```python
from build123d import *

# Parameters (mm, degrees)
BOSS_EXTRUDE1_DEPTH = 3
CUT_EXTRUDE3_DEPTH  = 10


with BuildPart() as part:
    # Sketch1 → Boss-Extrude1 (new body)
    with BuildSketch(Plane.XY):
        Polygon((-41.404007678, -45.884292091), (30.844012981, -53.556577334), (60.46665605, 12.784506978), (6.526435644, 61.457837175), (-56.433096997, 25.198525272), align=None)
    extrude(amount=BOSS_EXTRUDE1_DEPTH)

    # Sketch4 → Cut-Extrude3 (cut)
    with BuildSketch(Plane.XY.offset(3)):
        Polygon((-50.814192878, 22.62393629), (-39.77384321, 28.998085143), (-42.284603166, 33.346848953), (-56.433096997, 25.198525272), (-53.055705701, 9.224537525), (-48.18384365, 10.249116114), align=None)
        Polygon((5.814192878, 55.31835005), (15.288024352, 46.788073876), (18.648077016, 50.519790415), (6.526435644, 61.457837175), (-7.622058187, 53.309513494), (-5.142137875, 48.99270954), align=None)
        Polygon((54.407561694, 11.564684243), (49.22236188, -0.08146522), (53.809748587, -2.123901372), (60.46665605, 12.784506978), (48.345014677, 23.722553738), (45.005827668, 20.030043583), align=None)
        Polygon((37.500920444, -38.648168984), (32.957269066, -36.61346181), (27.811529494, -48.170982119), (15.133068296, -46.838422151), (14.608176536, -51.832433652), (30.844012981, -53.556577334), align=None)
        Polygon((-25.168171234, -47.608435773), (-24.637115209, -42.658407427), (-37.219091188, -41.335988464), (-39.869611319, -28.866271649), (-44.781398973, -29.910304344), (-41.404007678, -45.884292091), align=None)
    extrude(amount=-CUT_EXTRUDE3_DEPTH, mode=Mode.SUBTRACT)


solid = part.part
```
Here's how the part is built. I have some questions about the finished solid (model axes, mm). A direction names the side the tool comes from. Round coordinates to 2 decimals unless told otherwise and drop trailing zeros. Loops run counter-clockwise (first coordinate to the right, second up) from the corner with the lowest first, then second, coordinate; pieces in that order, holes last. Notation, with made-up numbers: (-17.5, 58) -> (-9.5, 58) arc R29 ccw to (-9.5, 84) -> close; hole circle Ø5 at (1.25, -12.5). An arc over 180 degrees is marked (long way). Answer as CSV lines item,"result".
1. Thinking about a two-plate mould opening in X: for faces 6 (the face through (0, 2, 0)), 7 (the face through (-49.48, 16.35, 1.52)), 8 (the face through (10.5, 51.1, 1.5)), 9 (the face through (46.699, 21.902, 1.521)), which applies, released by +X, released by -X, zero draft, split by the parting line, or undercut?
Final values:
face 6,"zero draft"
face 7,"released by -X"
face 8,"undercut"
face 9,"released by +X"
2. If I drill on L1, parallel to Y at x = -40, z = 1.9; L2, parallel to Y at x = 46, z = 1.85; L3, parallel to X at y = -38, z = 0.3, over which ranges is the centre line in solid material (lowest first)?
Final values:
L1,"y = -28.89 to 28.87, 29.39 to 34.66"
L2,"y = -19.61 to 19.13, 21.13 to 25.84"
L3,"x = -37.93 to 32.34, 36.05 to 37.79"
3. Which directions (+Z, -Z, +X, -X, +Y, -Y) give clear straight access to the entire face, cutting with the end or side of a thin tool? Please do faces 1 (the face through (49.64, 15.86, 1.52)), 2 (the face through (0, 2, 3)), 3 (the face through (-6.4, 51.18, 1.52)), 4 (the face through (-42.29, -29.38, 1.52)), 5 (the face through (-41.01, 31.14, 1.52)).
Final values:
face 1,"+Z, -Z, +X"
face 2,"+Z, +X, -X, +Y, -Y"
face 3,"+Z, -Z, +Y"
face 4,"+Z, -Z, -Y"
face 5,"+Z, -Z, -X"
4. For pin 1 (1.5 mm diameter, centred on y = 12.5, z = 2, fed in from -X); pin 2 (1 mm diameter, centred on y = 20.5, z = 2.5, fed in from +X); pin 3 (1 mm diameter, centred on x = -17.5, z = 2, fed in from +Y), each with a flat end and sliding along its axis, tell me the tip position at first contact or that it passes through.
Final values:
pin 1,"stops at x = -48.82"
pin 2,"stops at x = 45.88"
pin 3,"stops at y = 47.91"
5. If we section it at B-B on x = 30: Please give me the cut outline in (y, z), plus the area to 3 significant figures.
Final values:
outline,"(-43.26, 0) -> (40.28, 0) -> (40.28, 3) -> (-43.26, 3) -> close"
area,"251 mm^2"
6. If we section it at A-A on z = 1.05: Please give me the cut outline in (x, y).
Final values:
outline,"(-53.06, 9.22) -> (-44.78, -29.91) -> (-39.87, -28.87) -> (-37.22, -41.34) -> (-24.64, -42.66) -> (-25.17, -47.61) -> (14.61, -51.83) -> (15.13, -46.84) -> (27.81, -48.17) -> (32.96, -36.61) -> (37.5, -38.65) -> (53.81, -2.12) -> (49.22, -0.08) -> (54.41, 11.56) -> (45.01, 20.03) -> (48.35, 23.72) -> (18.65, 50.52) -> (15.29, 46.79) -> (5.81, 55.32) -> (-5.14, 48.99) -> (-7.62, 53.31) -> (-42.28, 33.35) -> (-39.77, 29) -> (-50.81, 22.62) -> (-48.18, 10.25) -> close"
7. If we section it at C-C on y = 42: Please give me the cut outline in (x, z), plus the area to 3 significant figures.
Final values:
outline,"(-27.26, 0) -> (28.09, 0) -> (28.09, 3) -> (-27.26, 3) -> close"
area,"166 mm^2"
